```python
from build123d import *

# Parameters (mm, degrees)
EXTRUDE_1_DEPTH = 170
FILLET_1_R      = 1


with BuildPart() as part:
    # 草图1 → 凸台-拉伸1 (new body)
    with BuildSketch(Plane.XY):
        with BuildLine():
            Line((0, 0), (25, 0))
            Line((25, 0), (25, 2))
            Line((25, 2), (7, 2))
            ThreePointArc((7, 2), (3.464466094, 3.464466094), (2, 7))
            Line((2, 7), (2, 25))
            Line((2, 25), (0, 25))
            Line((0, 25), (0, 0))
        make_face()
    extrude(amount=EXTRUDE_1_DEPTH)

    # 圆角1
    fillet_1_edges = [part.edges().sort_by_distance(p)[0] for p in [
        (0, 25, 85),
        (25, 2, 85),
        (25, 0, 85),
        (0, 0, 85),
        (2, 25, 85),
    ]]
    fillet(fillet_1_edges, radius=FILLET_1_R - 0.0001)  # a hair under: the kernel refuses the full size


solid = part.part
```
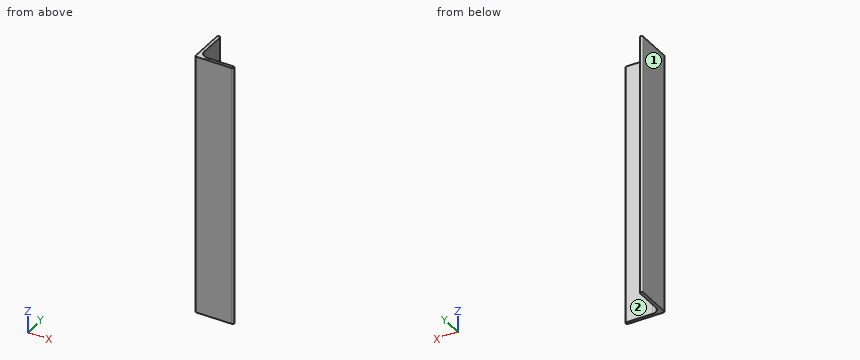
Read the model definition and answer for the solid it produces. Units are mm, in the model's axes. Face numbers are marked on the shaded views. A direction names the side the tool comes from. Give positions to 0.01 mm unless a question says otherwise; leave off trailing zeros. Write each loop counter-clockwise with the first axis right and the second up, starting at its lowest first coordinate (ties: lowest second). Pieces come first, ordered by that corner, then holes. Notation, with made-up numbers: M -29.5,89.5 L 14.5,89.5 A18 ccw 14.5,124.5 Z; hole C 25.5,11.5 d2. An arc over 180 degrees is marked long. Put each result on its own line as item: value. Start each with the question number.
1. Consider line 1 along Y through (x, z) = (13.75, 83.5); line 2 along Y through (x, z) = (4, 33.5). Determine where each line is inside the solid, lowest interval first.
2. The part is cut by section B-B, the plane x = 17.75. Give the vertices of the cut face in (y, z).
3. Each of these flat-tipped pins is pushed along its axis until it touches: pin 1 Ø2 at (x, z) = (9.5, 60.5) entering from +Y; pin 2 Ø4 at (y, z) = (5.5, 39) entering from +X; pin 3 Ø4 at (y, z) = (6.5, 147) entering from +X. Where does it stop, or does it pass through?
4. Which of the six approach directions +Z, -Z, +X, -X, +Y, -Y give full straight-line access (tool end or side, diameter ignored) to the marked faces 1 and 2?
Final values:
1. line 1: y = 0 to 2
1. line 2: y = 0 to 3
2. outline: M 0,0 L 2,0 L 2,170 L 0,170 Z
3. pin 1: stops at y = 2
3. pin 2: stops at x = 3.43
3. pin 3: stops at x = 2.67
4. face 1: +Z, -Z, -X, +Y, -Y
4. face 2: +Z, -Z, +X, +Y
